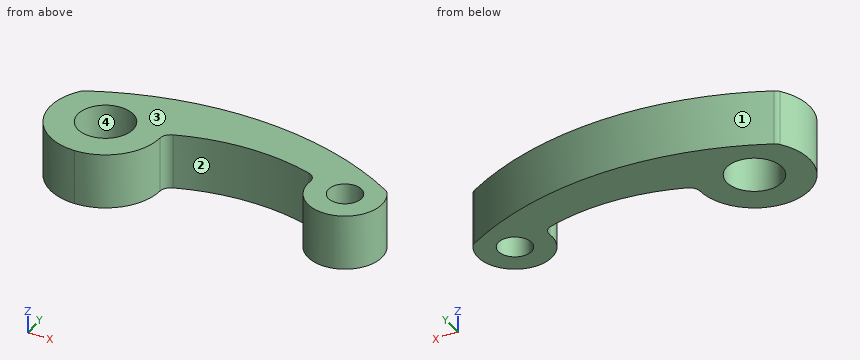
from build123d import *

# Parameters (mm, degrees)
F0_R     = 12.5
F0_R_2   = 7.5
F1_DEPTH = 25


with BuildPart() as f1:
    # F0 (on Top) → F1 (new body)
    with BuildSketch(Plane.XY):
        with BuildLine():
            ThreePointArc((-75.207108, 50.513876), (-76.212982, 49.861177), (-77.034532, 48.987763))
            ThreePointArc((-77.034532, 48.987763), (-79.21274, 22.88653), (-56.901976, 9.16615))
            ThreePointArc((-56.901976, 9.16615), (-39.216747, 16.496044), (-31.901986, 34.187538))
            ThreePointArc((-31.901986, 34.187538), (-31.012413, 37.038638), (-28.656223, 38.873979))
            ThreePointArc((-28.656223, 38.873979), (1.960124, 44.874089), (32.869195, 40.632465))
            ThreePointArc((32.869195, 40.632465), (35.523586, 38.663847), (36.370146, 35.469386))
            ThreePointArc((36.370146, 35.469386), (57.04258, 17.857846), (67.38122, 42.970162))
            ThreePointArc((67.38122, 42.970162), (66.636188, 43.906127), (65.690151, 44.638329))
            ThreePointArc((65.690151, 44.638329), (-4.012921, 65.454779), (-75.207108, 50.513876))
        make_face()
        with Locations((-56.901976, 34.16615)):
            Circle(F0_R, mode=Mode.SUBTRACT)
        with Locations((53.098024, 34.16615)):
            Circle(F0_R_2, mode=Mode.SUBTRACT)
    extrude(amount=F1_DEPTH)


solid = f1.part
The model under review builds one solid part; all positions refer to its coordinate system, in mm. Face numbers are marked on the shaded views. Give positions to 0.01 mm unless a question says otherwise; leave off trailing zeros. Loops run counter-clockwise (first coordinate to the right, second up) from the corner with the lowest first, then second, coordinate; pieces in that order, holes last. Notation, with made-up numbers: (62.5, 17) -> (81.5, 17) arc R26 cw to (81.5, 36) -> close; hole circle Ø8 at (43.25, 45.25). An arc over 180 degrees is marked (long way). Write each question's results on one line, items separated by ' | '.
1) Take a section at C-C, the plane z = 14.25. Give the boundary of the cut face in (x, y), plus the area to 3 significant figures.
Conclusion:
outline: (-77.03, 48.99) arc R25 ccw (long way) to (-31.9, 34.19) arc R5 cw to (-28.66, 38.87) arc R95 cw to (32.87, 40.63) arc R5 cw to (36.37, 35.47) arc R16.78 ccw (long way) to (67.38, 42.97) arc R5 ccw to (65.69, 44.64) arc R147.86 ccw to (-75.21, 50.51) arc R5 ccw to start; hole circle Ø25 at (-56.9, 34.17); hole circle Ø15 at (53.1, 34.17) | area: 3,870 mm^2
2) Insertion check: pin 1 Ø5 at (x, z) = (51, 6) entering from +Y; pin 2 Ø8 at (y, z) = (23, 22) entering from -X; pin 3 Ø1.5 at (y, z) = (32.5, 11.5) entering from +X. Each pin has a flat end and moves straight along its axis. Give the tip position at first contact, or say it passes through.
Conclusion:
pin 1: stops at y = 53.44 | pin 2: stops at x = -80.85 | pin 3: stops at x = 69.85
3) Take a section at A-A, the plane x = 55.5. Give the boundary of the cut face in (y, z).
Conclusion:
outline: (17.56, 0) -> (27.06, 0) -> (27.06, 25) -> (17.56, 25) -> close; (41.27, 0) -> (50.2, 0) -> (50.2, 25) -> (41.27, 25) -> close
4) Take a section at B-B, the plane y = 29. Give the boundary of the cut face in (x, z).
Conclusion:
outline: (-81.36, 0) -> (-68.28, 0) -> (-68.28, 25) -> (-81.36, 25) -> close; (-45.52, 0) -> (-32.44, 0) -> (-32.44, 25) -> (-45.52, 25) -> close; (37.13, 0) -> (47.66, 0) -> (47.66, 25) -> (37.13, 25) -> close; (58.54, 0) -> (69.06, 0) -> (69.06, 25) -> (58.54, 25) -> close
5) Take a section at D-D, the plane x = 14. Give the boundary of the cut face in (y, z).
Conclusion:
outline: (44.45, 0) -> (63.59, 0) -> (63.59, 25) -> (44.45, 25) -> close
6) Draft analysis for pull direction Y (two halves, no side actions). For the marked faces 1, 2, 3 and 4, state which applies: pulls with the +Y half, pulls with the -Y half, needs draft (parallel to the pull), parting line crosses it, or undercut.
Conclusion:
face 1: pulls with the +Y half | face 2: pulls with the -Y half | face 3: needs draft | face 4: undercut
7) For line 1 along X through (y, z) = (34, 21.75); line 2 along X through (y, z) = (24, 23); line 3 along X through (y, z) = (31.5, 19.5), list the stretches that pass through material, from the lowest coordinate up. Write a range as from..to.
Conclusion:
line 1: x = -81.9..-69.4, -44.4..-31.9, 36.32..45.6, 60.6..69.88 | line 2: x = -79.74..-64.18, -49.63..-34.06, 39.75..66.45 | line 3: x = -81.76..-69.11, -44.69..-32.04, 36.53..46.09, 60.11..69.66
